Part print with two shaded views. Sizes in mm from the minimum x, y, z corner. A direction names the side the tool comes from. Round coordinates to 2 decimals unless told otherwise and drop trailing zeros. Order: outer loops, then holes, each group sorted by start corner. A loop starts at its lowest first (then second) coordinate and runs counter-clockwise, first axis right, second up. Notation, with made-up numbers: M 4,-1.75 L 29,-1.75 A23 ccw 29,37.25 Z; hole C -36,-29 d11. An arc over 180 degrees is marked long. Put each result on its own line as item: value.
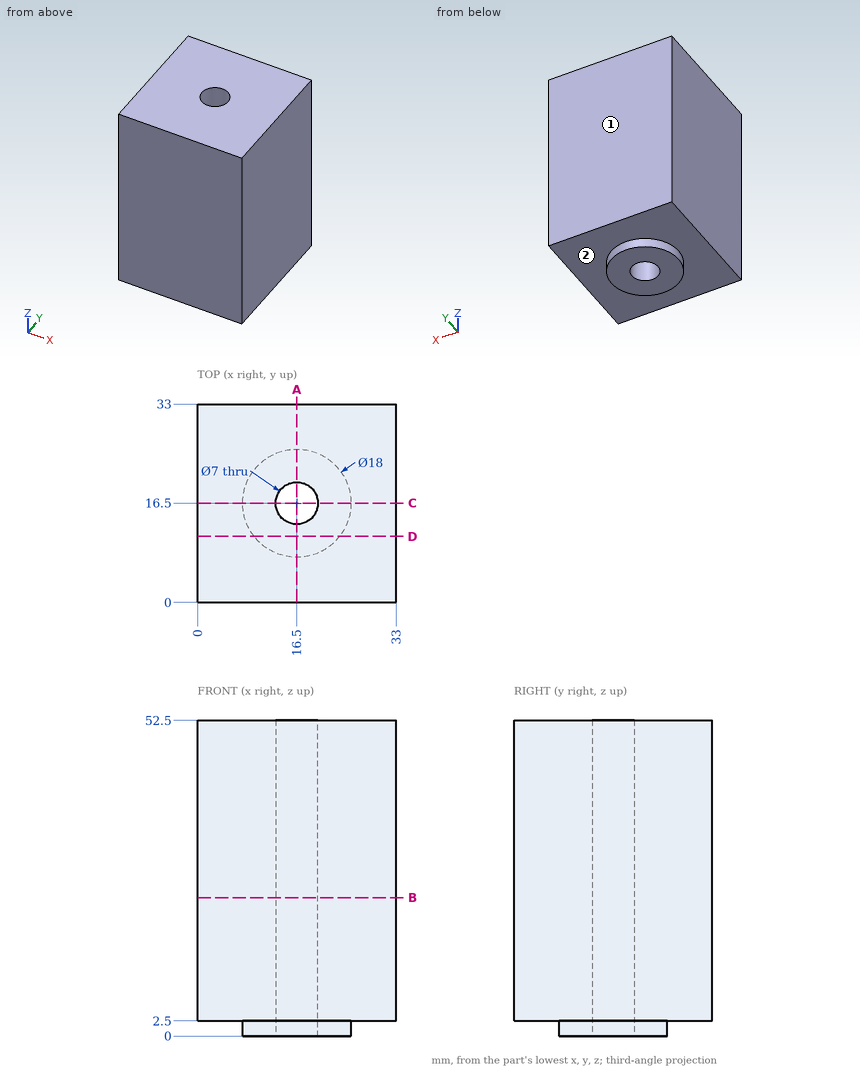
Item 1: Band-saw the part on D-D on y = 11. Give the cut face in (x, z), and give its area (3 significant figures).
Answers below:
outline: M 0,2.5 L 9.38,2.5 L 9.38,0 L 23.62,0 L 23.62,2.5 L 33,2.5 L 33,52.5 L 0,52.5 Z
area: 1,690 mm²
Item 2: Band-saw the part on B-B on z = 23. Give the cut face in (x, y), and give its area (3 significant figures).
Answers below:
outline: M 0,0 L 33,0 L 33,33 L 0,33 Z; hole C 16.5,16.5 d7
area: 1,050 mm²
Item 3: Tool access for the marked faces 1 and 2: list every direction of +Z, -Z, +X, -X, +Y, -Y with a clear straight run to the whole face (end or side of a thin tool).
Answers below:
face 1: +Z, -Z, +X, -X, +Y
face 2: -Z
Item 4: Probe line 1 along X through (y, z) = (16.5, 42); line 2 along Z through (x, y) = (9, 8). List the from-to ranges inside material, lowest first. Write a range as [from, to].
Answers below:
line 1: [0, 13], [20, 33]
line 2: [2.5, 52.5]
Item 5: Pin check, flat tip, straight feed: P1, Ø4, axis at x = 28.5, y = 15, coming from the -Z side. Stop position of the tip, or through.
Answers below:
P1: z = 2.5
Item 6: Band-saw the part on A-A on x = 16.5. Give the cut face in (y, z).
Answers below:
outline: M 0,2.5 L 7.5,2.5 L 7.5,0 L 13,0 L 13,52.5 L 0,52.5 Z; M 20,0 L 25.5,0 L 25.5,2.5 L 33,2.5 L 33,52.5 L 20,52.5 Z
